```python
from build123d import *

# Parameters (mm, degrees)
EXTRUDE1_START              = -54
SKETCH1_R                   = 7.9375
EXTRUDE1_DEPTH              = 54
EXTRUDE4_DEPTH              = 4
F_3_8_24_TAPPED_HOLE1_D     = 8.4328
F_3_8_24_TAPPED_HOLE1_DEPTH = 24.35
F_3_8_24_TAPPED_HOLE1_TIP   = 2.533468714


with BuildPart() as part:
    # Sketch1 → Extrude1 (new body)
    with BuildSketch(Plane(origin=(0, 0, 0), x_dir=(1, 0, 0), z_dir=(0, 1, 0)).offset(EXTRUDE1_START)):
        Circle(SKETCH1_R)
    extrude(amount=EXTRUDE1_DEPTH)

    # Sketch4 → Extrude4 (add)
    with BuildSketch(Plane.XZ.offset(54)):
        with BuildLine():
            Line((-7.82879301, 10), (7.82879301, 10))
            ThreePointArc((7.82879301, 10), (12.7, 0), (7.82879301, -10))
            Line((7.82879301, -10), (-7.82879301, -10))
            ThreePointArc((-7.82879301, -10), (-12.7, 0), (-7.82879301, 10))
        make_face()
    extrude(amount=EXTRUDE4_DEPTH)

    # 3_8-24 Tapped Hole1
    with Locations(Plane(origin=(0, 0, 0), x_dir=(-1, 0, 0), z_dir=(0, 1, 0))):
        with Locations((0, 0)):
            Hole(F_3_8_24_TAPPED_HOLE1_D / 2, depth=F_3_8_24_TAPPED_HOLE1_DEPTH)
            with Locations((0, 0, -(F_3_8_24_TAPPED_HOLE1_DEPTH + F_3_8_24_TAPPED_HOLE1_TIP / 2))):  # 118° drill point
                Cone(0, F_3_8_24_TAPPED_HOLE1_D / 2, F_3_8_24_TAPPED_HOLE1_TIP, mode=Mode.SUBTRACT)


solid = part.part
```
Source: CAD feature listing. Evaluate the final solid. Frame: model axes, mm. A direction names the side the tool comes from. Give positions to 0.01 mm unless a question says otherwise; leave off trailing zeros. Write each loop counter-clockwise with the first axis right and the second up, starting at its lowest first coordinate (ties: lowest second). Pieces come first, ordered by that corner, then holes. Notation, with made-up numbers: (88, 61.25) - (108, 61.25) arc R19 cw to (108, 93.25) - close; hole circle Ø4 at (86.25, 3.5). An arc over 180 degrees is marked (long way). One line per item, written item: value. Start each with the question number.
Q1. Section query C-C, the plane y = -35.5. Return the cut outline in (x, z) (1 decimal), then the cut area to 3 significant figures.
Q2. Section query D-D, the plane y = -25. Return the cut outline in (x, z) (1 decimal), then the cut area to 3 significant figures.
Q3. Draft query along X for faces 1 (the face through (-0.55, -12.35, 4.18)), 2 (the face through (0, -58, 0)), 3 (the face through (-1.72, -27.38, 7.75)). Return one class per face: +X half, -X half, draft (parallel to the pull), parting line (faces both ways), or undercut.
Q4. First-contact query: pin 1 Ø4 at (x, y) = (-1.5, -18.5) entering from -Z; pin 2 Ø6 at (x, z) = (-2.5, 2) entering from +Y; pin 3 Ø1 at (x, y) = (3, -7.5) entering from -Z; pin 4 Ø8 at (x, y) = (-10, -29.5) entering from -Z. Flat tips, straight axial feed; report the tip coordinate or a pass-through.
Q5. Section query B-B, the plane x = -6.25. Return the cut outline in (y, z), then the cut area to 3 significant figures.
Q6. Material intervals for probe 1 along Z at (x, y) = (0, -16.5); probe 2 along Y at (x, z) = (10.75, 3), sorted ascending. Write a range as from..to.
Q7. Section query A-A, the plane y = -6. Return the cut outline in (x, z) (1 decimal), then the cut area to 3 significant figures.
Q8. Set-up query: faces 4 (the face through (0, -56, -10)), 5 (the face through (-8.3, -54, 0.1)). Return all of +Z, -Z, +X, -X, +Y, -Y with unobstructed straight access to the full face (end or side cutting, diameter ignored); none if empty.
Answer:
1. outline: circle Ø15.9 at (0, 0)
1. area: 198 mm2
2. outline: circle Ø15.9 at (0, 0); hole circle Ø6.3 at (0, 0)
2. area: 167 mm2
3. face 1: undercut
3. face 2: draft
3. face 3: parting line
4. pin 1: stops at z = -7.94
4. pin 2: stops at y = 0
4. pin 3: stops at z = -7.53
4. pin 4: stops at z = -5.2
5. outline: (-58, -10) - (-54, -10) - (-54, -4.89) - (0, -4.89) - (0, 4.89) - (-54, 4.89) - (-54, 10) - (-58, 10) - close
5. area: 608 mm2
6. probe 1: z = -7.94..-4.22, 4.22..7.94
6. probe 2: y = -58..-54
7. outline: circle Ø15.9 at (0, 0); hole circle Ø8.4 at (0, 0)
7. area: 142 mm2
8. face 4: -Z, +X, -X, +Y, -Y
8. face 5: +Y
